```python
from build123d import *

# Parameters (mm, degrees)
SKETCH1_R                = 11.25
SKETCH1_R_2              = 3
BOSS_EXTRUDE1_DEPTH      = 3
BOSS_EXTRUDE2_DEPTH      = 3
FILLET1_R                = 0.25
CIRPATTERN1_COUNT        = 17
FILLET1_OF_CIRPATTERN1_R = 0.25
BOSS_EXTRUDE3_START      = -3.5
SKETCH3_R                = 5
SKETCH3_R_2              = 3
BOSS_EXTRUDE3_DEPTH      = 3.5


with BuildPart() as part:
    # Sketch1 → Boss-Extrude1 (new body)
    with BuildSketch(Plane.XY):
        Circle(SKETCH1_R)
        Circle(SKETCH1_R_2, mode=Mode.SUBTRACT)
    extrude(amount=BOSS_EXTRUDE1_DEPTH)

    # Sketch2 → Boss-Extrude2 (add)
    with BuildSketch(Plane.XY):
        Polygon((-1.323267478, 10.75), (-1.323267478, 11.55), (-0.625, 14.25), (0.625, 14.25), (1.323267478, 11.55), (1.323267478, 10.75), align=None)
    boss_extrude2 = extrude(amount=BOSS_EXTRUDE2_DEPTH)

    # Fillet1
    fillet1_edges = [part.edges().sort_by_distance(p)[0] for p in [
        (0.625, 14.25, 1.5),
        (-0.625, 14.25, 1.5),
    ]]
    fillet(fillet1_edges, radius=FILLET1_R)

    # CirPattern1: Boss-Extrude2 ×17 about axis
    cirpattern1_axis = Axis((0, 0, 0), (0, 0, 1))
    for i in range(1, CIRPATTERN1_COUNT):
        add(boss_extrude2.rotate(cirpattern1_axis, i * 360 / CIRPATTERN1_COUNT))

    # Fillet1 of CirPattern1
    fillet1_of_cirpattern1_edges = [part.edges().sort_by_distance(p)[0] for p in [
        (-4.5648986, 13.51350531, 1.5),
        (-5.730488887, 13.061953228, 1.5),
        (-9.138282349, 10.951936848, 1.5),
        (-10.062043495, 10.109817293, 1.5),
        (-12.477490429, 6.911248627, 1.5),
        (-13.034663374, 5.792294513, 1.5),
        (-14.131544288, 1.937157983, 1.5),
        (-14.246879737, 0.692490262, 1.5),
        (-13.877054784, -3.298556582, 1.5),
        (-13.534976046, -4.500838636, 1.5),
        (-11.748392136, -8.088782801, 1.5),
        (-10.995098841, -9.086304335, 1.5),
        (-8.033044031, -11.786574082, 1.5),
        (-6.970272611, -12.444614286, 1.5),
        (-3.232788816, -13.892523222, 1.5),
        (-2.004072442, -14.122210119, 1.5),
        (2.004072442, -14.122210119, 1.5),
        (3.232788816, -13.892523222, 1.5),
        (6.970272611, -12.444614286, 1.5),
        (8.033044031, -11.786574082, 1.5),
        (10.995098841, -9.086304335, 1.5),
        (11.748392136, -8.088782801, 1.5),
        (13.534976046, -4.500838636, 1.5),
        (13.877054784, -3.298556582, 1.5),
        (14.246879737, 0.692490262, 1.5),
        (14.131544288, 1.937157983, 1.5),
        (13.034663374, 5.792294513, 1.5),
        (12.477490429, 6.911248627, 1.5),
        (10.062043495, 10.109817293, 1.5),
        (9.138282349, 10.951936848, 1.5),
        (5.730488887, 13.061953228, 1.5),
        (4.5648986, 13.51350531, 1.5),
    ]]
    fillet(fillet1_of_cirpattern1_edges, radius=FILLET1_OF_CIRPATTERN1_R)

    # Sketch3 → Boss-Extrude3 (add)
    with BuildSketch(Plane.XY.offset(BOSS_EXTRUDE3_START)):
        Circle(SKETCH3_R)
        Circle(SKETCH3_R_2, mode=Mode.SUBTRACT)
    extrude(amount=BOSS_EXTRUDE3_DEPTH)


solid = part.part
```
CAD build for the part. Positions are in the model's coordinates, mm. A direction names the side the tool comes from. Coordinates: 2 decimals unless noted, no trailing zeros. Loops run counter-clockwise (first coordinate to the right, second up) from the corner with the lowest first, then second, coordinate; pieces in that order, holes last. Notation, with made-up numbers: (-3, 2) - (20, 2) arc R24 cw to (20, 14) - close; hole circle Ø8 at (-19, -27). An arc over 180 degrees is marked (long way). Return JSON: item names as keys, results as strings.
1. Band-saw the part on C-C (x = 3.75). Give the cut face in (y, z), and give its area (3 significant figures).
Result:
{"outline": "(-10.61, 0) - (-3.31, 0) - (-3.31, -3.5) - (3.31, -3.5) - (3.31, 0) - (12.38, 0) - (12.38, 3) - (-10.61, 3) - close", "area": "92.1 mm2"}
2. Band-saw the part on D-D (y = 8.75). Give the cut face in (x, z), and give its area (3 significant figures).
Result:
{"outline": "(-9.34, 0) - (9.34, 0) - (9.34, 3) - (-9.34, 3) - close", "area": "56.1 mm2"}
3. Probe L1, parallel to Y at x = 0, z = 1; L2, parallel to Y at x = 0, z = -0.25; L3, parallel to X at y = 12, z = 2. List the from-to ranges inside material, lowest first. Write a range as from..to.
Result:
{"L1": "y = -11.25..-3, 3..14.25", "L2": "y = -5..-3, 3..5", "L3": "x = -5.61..-3.48, -1.21..1.21, 3.48..5.61"}
4. 3-axis set-ups, long thin cutter, end or side, ignore diameter. For faces 4 (the flat face through (3.336, -12.387, 1.479)), 5 (the flat face through (12.861, 0.194, 1.479)), 6 (the flat face through (-5.555, 11.563, 1.479)), 7 (the flat face through (5.14, 13.29, 1.48)), 8 (the cylindrical face through (-1.08, -4.88, -1.77)): which of +Z, -Z, +X, -X, +Y, -Y reach the whole face in a straight line?
Result:
{"face 4": "+Z, -Z, -Y", "face 5": "+Z, -Z, +X", "face 6": "+Z, -Z", "face 7": "+Z, -Z, +X, +Y", "face 8": "-Z"}
5. Band-saw the part on B-B (z = -2.5). Give the cut face in (x, y), and give its area (3 significant figures).
Result:
{"outline": "circle Ø10 at (0, 0); hole circle Ø6 at (0, 0)", "area": "50.3 mm2"}
6. Drop a flat-ended pin along its axis: pin 1 (1 mm diameter, centred on x = 5, z = -2.5, fed in from -Y). Give the stop position or say it passes through.
Result:
{"pin 1": "stops at y = -2.18"}
7. Mould opens along X. For faces 1 (the flat face through (-2.61, -14.01, 1.48)), 2 (the flat face through (13.71, -3.89, 1.48)), 3 (the flat face through (9.63, -8.52, 1.48)) say: released by +X, released by -X, zero draft, split by the parting line, or undercut.
Result:
{"face 1": "released by -X", "face 2": "released by +X", "face 3": "undercut"}
8. Band-saw the part on A-A (x = 0). Give the cut face in (y, z), and give its area (3 significant figures).
Result:
{"outline": "(-11.25, 0) - (-5, 0) - (-5, -3.5) - (-3, -3.5) - (-3, 3) - (-11.25, 3) - close; (3, -3.5) - (5, -3.5) - (5, 0) - (14.25, 0) - (14.25, 3) - (3, 3) - close", "area": "72.5 mm2"}
